Input: dimensioned drawing with shaded views. Units: mm. Origin: part minimum x, y, z. A direction names the side the tool comes from. Give positions to 0.01 mm unless a question says otherwise; leave off trailing zeros. Loops run counter-clockwise (first coordinate to the right, second up) from the corner with the lowest first, then second, coordinate; pieces in that order, holes last.
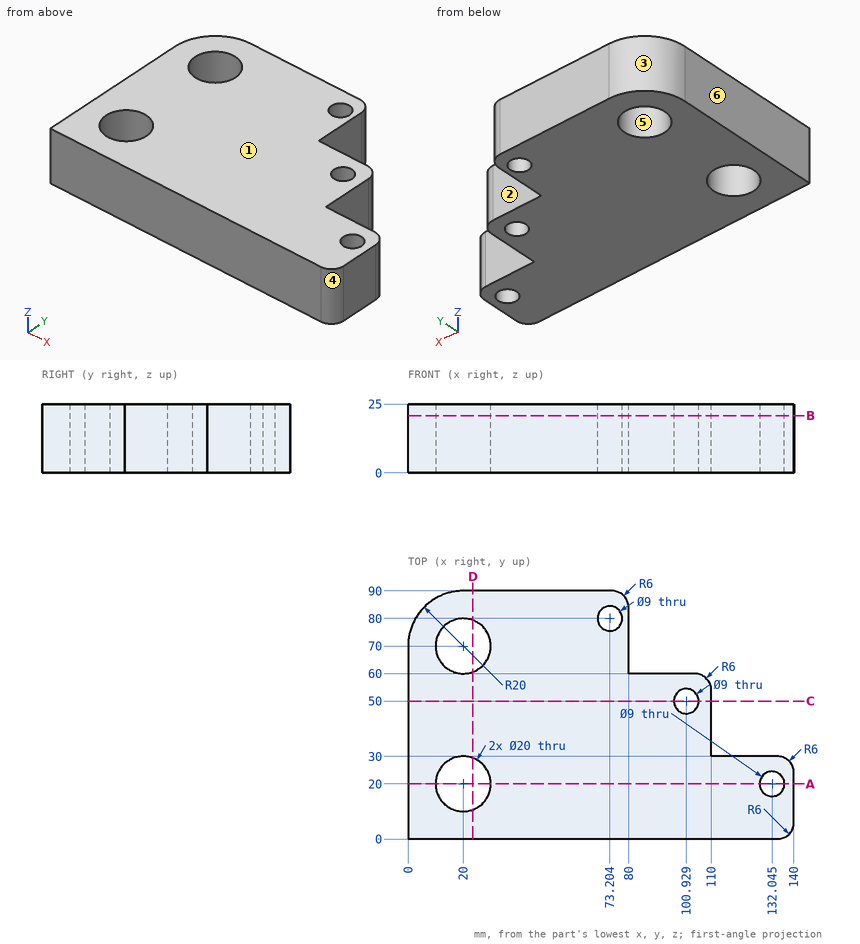
Item 1: Draft query along Y for the marked faces 3, 4, 5 and 6. Return one class per face: +Y half, -Y half, draft (parallel to the pull), parting line (faces both ways), or undercut.
Values follow:
face 3: +Y half
face 4: -Y half
face 5: undercut
face 6: draft
Item 2: Pin query (flat end, axial travel): pin 1 (7 mm diameter, centred on y = 70, z = 7.5, fed in from +X); pin 2 (6 mm diameter, centred on y = 29.5, z = 14.5, fed in from +X) (1 decimal); pin 3 (12 mm diameter, centred on x = 120.5, z = 10, fed in from +Y). Return the tip coordinate at first contact, or that it passes through.
Values follow:
pin 1: stops at x = 80
pin 2: stops at x = 139.5
pin 3: stops at y = 30
Item 3: Ray query, probe 1 along Y at (x, z) = (20, 19.5); probe 2 along Y at (x, z) = (13, 23.25) (1 decimal); probe 3 along X at (y, z) = (16.5, 23) (1 decimal). Return the intervals inside material, ascending.
Values follow:
probe 1: y = 0 to 10, 30 to 60, 80 to 90
probe 2: y = 0 to 12.9, 27.1 to 62.9, 77.1 to 88.7
probe 3: x = 0 to 10.6, 29.4 to 129.2, 134.9 to 140
Item 4: Section query B-B on z = 20.75. Return loops of the section in (x, y) (1 decimal), plus the area to 3 significant figures.
Values follow:
outline: (0, 0) - (134, 0) arc R6 ccw to (140, 6) - (140, 24) arc R6 ccw to (134, 30) - (110, 30) - (110, 54) arc R6 ccw to (104, 60) - (80, 60) - (80, 84) arc R6 ccw to (74, 90) - (20, 90) arc R20 ccw to (0, 70) - close; hole circle Ø20 at (20, 20); hole circle Ø20 at (20, 70); hole circle Ø9 at (73.2, 80); hole circle Ø9 at (100.9, 50); hole circle Ø9 at (132, 20)
area: 8,960 mm2
Item 5: Section query A-A on y = 20. Return loops of the section in (x, z) (1 decimal), plus the area to 4 significant figures.
Values follow:
outline: (0, 0) - (10, 0) - (10, 25) - (0, 25) - close; (30, 0) - (127.5, 0) - (127.5, 25) - (30, 25) - close; (136.5, 0) - (140, 0) - (140, 25) - (136.5, 25) - close
area: 2,775 mm2
Item 6: Section query D-D on x = 23.5. Return loops of the section in (y, z), plus the area to 3 significant figures.
Values follow:
outline: (0, 0) - (10.63, 0) - (10.63, 25) - (0, 25) - close; (29.37, 0) - (60.63, 0) - (60.63, 25) - (29.37, 25) - close; (79.37, 0) - (90, 0) - (90, 25) - (79.37, 25) - close
area: 1,310 mm2
Item 7: Section query C-C on y = 50. Return loops of the section in (x, z).
Values follow:
outline: (0, 0) - (96.43, 0) - (96.43, 25) - (0, 25) - close; (105.43, 0) - (110, 0) - (110, 25) - (105.43, 25) - close
Item 8: Set-up query: the marked faces 1 and 2. Return all of +Z, -Z, +X, -X, +Y, -Y with unobstructed straight access to the full face (end or side cutting, diameter ignored); none if empty.
Values follow:
face 1: +Z, +X, -X, +Y, -Y
face 2: +Z, -Z, +X, +Y
